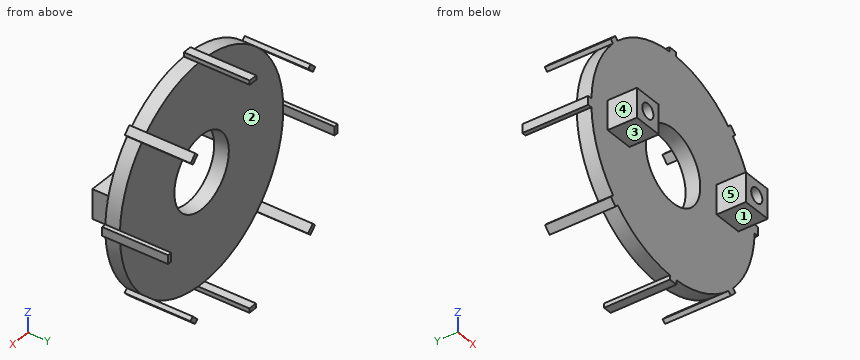
```python
from build123d import *

# Parameters (mm, degrees)
SKETCH1_R           = 75
BOSS_EXTRUDE1_DEPTH = 10
SKETCH2_R           = 25
CUT_EXTRUDE1_DEPTH  = 10
SKETCH3_W           = 20
SKETCH3_H           = 20
BOSS_EXTRUDE2_DEPTH = 20
SKETCH4_R           = 5.1
CUT_EXTRUDE2_DEPTH  = 20
SKETCH5_W           = 6
SKETCH5_H           = 3.326162104
SKETCH5_W_2         = 3.326162104
SKETCH5_H_2         = 6
BOSS_EXTRUDE3_DEPTH = 10
SKETCH6_W           = 2.933357957
SKETCH6_H           = 6
BOSS_EXTRUDE4_DEPTH = 35


with BuildPart() as part:
    # Sketch1 → Boss-Extrude1 (new body)
    with BuildSketch(Plane(origin=(0, 0, 0), x_dir=(1, 0, 0), z_dir=(0, 1, 0))):
        with Locations(Location((0, 0, 0), (0, 0, 270))):
            Circle(SKETCH1_R)
    extrude(amount=BOSS_EXTRUDE1_DEPTH)

    # Sketch2 → Cut-Extrude1 (cut)
    with BuildSketch(Plane(origin=(0, 10, 0), x_dir=(1, 0, 0), z_dir=(0, 1, 0))):
        with Locations(Location((0, 0, 0), (0, 0, 270))):
            Circle(SKETCH2_R)
    extrude(amount=-CUT_EXTRUDE1_DEPTH, mode=Mode.SUBTRACT)

    # Sketch3 → Boss-Extrude2 (add)
    with BuildSketch(Plane.XZ):
        with Locations((50, 0)):
            Rectangle(SKETCH3_W, SKETCH3_H)
        with Locations((-50, 0)):
            Rectangle(SKETCH3_W, SKETCH3_H)
    extrude(amount=BOSS_EXTRUDE2_DEPTH)

    # Sketch4 → Cut-Extrude2 (cut)
    with BuildSketch(Plane.XZ.offset(20)):
        with Locations(Location((-50, 0, 0), (0, 0, 270))):
            Circle(SKETCH4_R)
        with Locations(Location((50, 0, 0), (0, 0, 270))):
            Circle(SKETCH4_R)
    extrude(amount=-CUT_EXTRUDE2_DEPTH, mode=Mode.SUBTRACT)

    # Sketch5 → Boss-Extrude3 (add)
    with BuildSketch(Plane(origin=(0, 10, 0), x_dir=(1, 0, 0), z_dir=(0, 1, 0))):
        Polygon((53.03387152, 57.087936355), (50.681919741, 54.735984576), (54.924560428, 50.493343889), (57.276512207, 52.845295668), align=None)
        with Locations((0.133343264, 76.204796053)):
            Rectangle(SKETCH5_W, SKETCH5_H)
        with Locations((76.204796053, -0.133343264)):
            Rectangle(SKETCH5_W_2, SKETCH5_H_2)
        Polygon((57.087936355, -53.03387152), (54.735984576, -50.681919741), (50.493343889, -54.924560428), (52.845295668, -57.276512207), align=None)
        with Locations((-0.133343264, -76.204796053)):
            Rectangle(SKETCH5_W, SKETCH5_H)
        Polygon((-53.03387152, -57.087936355), (-50.681919741, -54.735984576), (-54.924560428, -50.493343889), (-57.276512207, -52.845295668), align=None)
        with Locations((-76.204796053, 0.133343264)):
            Rectangle(SKETCH5_W_2, SKETCH5_H_2)
        Polygon((-57.087936355, 53.03387152), (-54.735984576, 50.681919741), (-50.493343889, 54.924560428), (-52.845295668, 57.276512207), align=None)
    extrude(amount=-BOSS_EXTRUDE3_DEPTH)

    # Sketch6 → Boss-Extrude4 (add)
    with BuildSketch(Plane(origin=(0, 10, 0), x_dir=(1, 0, 0), z_dir=(0, 1, 0))):
        Polygon((-2.866656736, 74.934519148), (0.128320094, 74.934519148), (0.133343264, 77.867877105), (-2.866656736, 77.867877105), (-2.866656736, 74.945195171), align=None)
        Polygon((0.133343264, 77.867877105), (0.128320094, 74.934519148), (3.133343264, 74.934519148), (3.133343264, 77.867877105), align=None)
        Polygon((-52.845295668, 57.276512207), (-57.087936355, 53.03387152), (-55.02128814, 50.967223305), (-55.013739052, 50.959674217), (-50.771098365, 55.202314904), align=None)
        Polygon((-57.276512207, -52.845295668), (-53.03387152, -57.087936355), (-50.967223305, -55.02128814), (-50.959674217, -55.013739052), (-55.202314904, -50.771098365), align=None)
        Polygon((-3.133343264, -77.867877105), (2.866656736, -77.867877105), (2.866656736, -74.945195171), (2.866656736, -74.934519148), (-3.133343264, -74.934519148), align=None)
        Polygon((52.845295668, -57.276512207), (57.087936355, -53.03387152), (55.02128814, -50.967223305), (55.013739052, -50.959674217), (50.771098365, -55.202314904), align=None)
        Polygon((77.867877105, -3.133343264), (77.867877105, 2.866656736), (74.945195171, 2.866656736), (74.934519148, 2.866656736), (74.934519148, -3.133343264), align=None)
        Polygon((57.276512207, 52.845295668), (53.03387152, 57.087936355), (50.967223305, 55.02128814), (50.959674217, 55.013739052), (55.202314904, 50.771098365), align=None)
        with Locations((-76.401198127, 0.133343264)):
            Rectangle(SKETCH6_W, SKETCH6_H)
    extrude(amount=BOSS_EXTRUDE4_DEPTH)


solid = part.part
```
Check sheet for the modelled part. Datum: model origin and axes. Units: mm. Face numbers are marked on the shaded views. A direction names the side the tool comes from. Coordinates: 2 decimals unless noted, no trailing zeros. Order: outer loops, then holes, each group sorted by start corner. A loop starts at its lowest first (then second) coordinate and runs counter-clockwise, first axis right, second up. Notation, with made-up numbers: (85.25, 38) -> (115.25, 38) arc R18 cw to (115.25, 57) -> close; hole circle Ø7 at (40.25, -27). An arc over 180 degrees is marked (long way). Write each question's results on one line, items separated by ' | '. Start each with the question number.
1) Section check A-A (y = -2.5). Enter the section's corners in (x, z), and give its area (3 significant figures).
2) Section check D-D (y = 32.5). Count the separate pieces of the cut face and the enclosed holes in it, and give its area (3 significant figures).
3) Material ranges on line 1 along X through (y, z) = (-7.5, 0); line 2 along Z through (x, y) = (-57, 3); line 3 along X through (y, z) = (3.75, 0), recorded low to high.
4) Draft check along X on the marked faces 3, 4 and 5. Enter one of: pulls with the +X half, pulls with the -X half, needs draft (parallel to the pull), parting line crosses it, or undercut.
5) Depth check by flat-ended pin: pin 1 (0.9 mm diameter, centred on x = 76.5, y = 27, fed in from +Z); pin 2 (3 mm diameter, centred on x = -50, z = -1.5, fed in from -Y); pin 3 (0.9 mm diameter, centred on y = 15, z = 76.5, fed in from -X). Enter the tip coordinate at first touch or a pass-through.
6) Section check C-C (x = 0). Enter the section's corners in (y, z), and give its area (3 significant figures).
7) Set-up check for the marked faces 1 and 2: record each of +Z, -Z, +X, -X, +Y, -Y from which the full face is reachable in a straight line by a thin tool's end or side.
8) Section check B-B (z = 0). Enter the section's corners in (x, y), and give its area (3 significant figures).
Checked values:
1) outline: (-60, -10) -> (-40, -10) -> (-40, 10) -> (-60, 10) -> close; (40, -10) -> (60, -10) -> (60, 10) -> (40, 10) -> close; hole circle Ø10.2 at (-50, 0); hole circle Ø10.2 at (50, 0) | area: 637 mm²
2) separate pieces: 8 | enclosed holes: 0 | area: 141 mm²
3) line 1: -60 to -55.1, -44.9 to -40, 40 to 44.9, 55.1 to 60 | line 2: -53.12 to -52.95, -48.74 to 48.74, 52.57 to 53.12 | line 3: -77.87 to -25, 25 to 77.87
4) face 3: needs draft | face 4: pulls with the -X half | face 5: undercut
5) pin 1: z = 3.13 | pin 2: y = 0 | pin 3: x = -3.13
6) outline: (0, -77.87) -> (45, -77.87) -> (45, -74.93) -> (10, -74.93) -> (10, -25) -> (0, -25) -> close; (0, 25) -> (10, 25) -> (10, 74.93) -> (45, 74.93) -> (45, 77.87) -> (0, 77.87) -> close | area: 1,260 mm²
7) face 1: -Z, +X, -X, -Y | face 2: +Y
8) outline: (-77.87, 0) -> (-60, 0) -> (-60, -20) -> (-55.1, -20) -> (-55.1, 0) -> (-44.9, 0) -> (-44.9, -20) -> (-40, -20) -> (-40, 0) -> (-25, 0) -> (-25, 10) -> (-74.93, 10) -> (-74.93, 45) -> (-77.87, 45) -> close; (25, 0) -> (40, 0) -> (40, -20) -> (44.9, -20) -> (44.9, 0) -> (55.1, 0) -> (55.1, -20) -> (60, -20) -> (60, 0) -> (77.87, 0) -> (77.87, 45) -> (74.93, 45) -> (74.93, 10) -> (25, 10) -> close | area: 1,650 mm²
